```python
from build123d import *

# Parameters (mm, degrees)
F0_W      = 13.2
F0_H      = 9.5
F1_DEPTH  = 7.9
F2_R      = 3
F3_DEPTH  = 8.8
F4_R      = 1.5
F5_DEPTH  = 11
F6_R      = 1.5
F7_W      = 2.424983
F7_H      = 0.470519
F7_W_2    = 2.78692
F7_H_2    = 0.398131
F8_DEPTH  = 4
F10_DEPTH = 1


with BuildPart() as f1:
    # F0 (on Right) → F1 (new body)
    with BuildSketch(Plane.YZ):
        with Locations((6.6, 4.75)):
            Rectangle(F0_W, F0_H)
    extrude(amount=F1_DEPTH)

    # F2 (on face) → F3 (join)
    with BuildSketch(Plane.XY.offset(9.5)):
        with Locations((3.95, 6.6)):
            Circle(F2_R)
    extrude(amount=F3_DEPTH)

    # F4 (on face) → F5 (join)
    with BuildSketch(Plane.XY.offset(18.3)):
        with Locations((3.95, 6.6)):
            Circle(F4_R)
    extrude(amount=F5_DEPTH)

    # F6
    f6_edges = [f1.edges().sort_by_distance(p)[0] for p in [
        (2.45, 6.6, 29.3),
    ]]
    fillet(f6_edges, radius=F6_R)

    # F7 (on face) → F8 (join)
    with BuildSketch(Plane(origin=(0, 0, 0), x_dir=(1, 0, 0), z_dir=(0, 0, -1))):
        with Locations((3.917066, -4.48028)):
            Rectangle(F7_W, F7_H)
        with Locations((4.025647, -10.090314)):
            Rectangle(F7_W_2, F7_H_2)
    extrude(amount=F8_DEPTH)

    # F9 (on face) → F10 (join)
    with BuildSketch(Plane.XY.offset(9.5)):
        Polygon((3.896882, 2.52701), (7.450754, 4.517503), (7.503872, 8.590493), (4.003118, 10.67299), (0.449246, 8.682497), (0.396128, 4.609507), align=None)
    extrude(amount=F10_DEPTH)


solid = f1.part
```
Geometry check sheet. Reference: the model listing, model coordinates, mm. A direction names the side the tool comes from. Coordinates: 2 decimals unless noted, no trailing zeros. Order: outer loops, then holes, each group sorted by start corner. A loop starts at its lowest first (then second) coordinate and runs counter-clockwise, first axis right, second up. Notation, with made-up numbers: (-36, 82.25) - (8, 82.25) arc R13 cw to (8, 89.25) - close; hole circle Ø2 at (76.5, -7.5). An arc over 180 degrees is marked (long way). Use one line per item in the form item = value.
1. Draft check along Y on faces 1 (the face through (2.122, 3.583, 9.993)), 2 (the face through (4, 9.891, -2)), 3 (the face through (1, 4, 9.5)), 4 (the face through (4, 7, 0)). Enter one of: pulls with the +Y half, pulls with the -Y half, needs draft (parallel to the pull), parting line crosses it, or undercut.
Here are the results:
face_1 = pulls with the -Y half
face_2 = undercut
face_3 = needs draft
face_4 = undercut
2. Scan lines: line 1 (Z direction, x = 4.5, y = 5); line 2 (Z direction, x = 5, y = 0.5); line 3 (Y direction, x = 3.75, z = 21). Record each from-to range of solid material in increasing order.
Here are the results:
line_1 = 0 to 18.3
line_2 = 0 to 9.5
line_3 = 5.11 to 8.09
3. Section check B-B (x = 3). Record the boundary of the cut face in (y, z), then the cut area to 3 significant figures.
Here are the results:
outline = (0, 0) - (4.25, 0) - (4.25, -4) - (4.72, -4) - (4.72, 0) - (9.89, 0) - (9.89, -4) - (10.29, -4) - (10.29, 0) - (13.2, 0) - (13.2, 9.5) - (10.11, 9.5) - (10.11, 10.5) - (9.45, 10.5) - (9.45, 18.3) - (7.76, 18.3) - (7.76, 27.8) arc R1.16 ccw to (5.44, 27.8) - (5.44, 18.3) - (3.75, 18.3) - (3.75, 10.5) - (3.06, 10.5) - (3.06, 9.5) - (0, 9.5) - close
area = 204 mm²
4. Gauge pin test, flat ends, axial feed: pin 1 (0.8 mm diameter, centred on x = 4, z = -1.5, fed in from -Y) (3 decimals); pin 2 (2 mm diameter, centred on x = 3, y = 8.5, fed in from +Z); pin 3 (2 mm diameter, centred on x = 7, y = 7, fed in from -Z). Record the tip position at first contact, or that the pin passes through.
Here are the results:
pin_1 = 4.245
pin_2 = 28.79
pin_3 = 0
5. Section check D-D (z = 27). Record the boundary of the cut face in (x, y), then the cut area to 3 significant figures.
Here are the results:
outline = circle Ø3 at (3.95, 6.6)
area = 7.07 mm²
6. Section check A-A (z = 10). Record the boundary of the cut face in (x, y).
Here are the results:
outline = (0.4, 4.61) - (3.9, 2.53) - (7.45, 4.52) - (7.5, 8.59) - (4, 10.67) - (0.45, 8.68) - close
7. Access from +Z, -Z, +X, -X, +Y, -Y to the whole of each face (thin tool, end or side, straight path). Record for faces 5 (the face through (6.81, 7.5, 14.35)), 6 (the face through (2.25, 9.69, 9.99)), 7 (the face through (4, 4.716, -2)).
Here are the results:
face_5 = +Z
face_6 = +Z, -X, +Y
face_7 = -Z, +X, -X
8. Section check C-C (y = 12.25). Record the boundary of the cut face in (x, z), then the cut area to 4 significant figures.
Here are the results:
outline = (0, 0) - (7.9, 0) - (7.9, 9.5) - (0, 9.5) - close
area = 75.05 mm²
